CAD build for the part. Positions are in the model's coordinates, mm. A direction names the side the tool comes from. Coordinates: 2 decimals unless noted, no trailing zeros. Loops run counter-clockwise (first coordinate to the right, second up) from the corner with the lowest first, then second, coordinate; pieces in that order, holes last. Notation, with made-up numbers: (15, 12.5) -> (74, 12.5) arc R13 cw to (74, 28.5) -> close; hole circle Ø3 at (-23, -18). An arc over 180 degrees is marked (long way). Answer as a JSON object with one key per item and string values. Group by question number.
from build123d import *

# Parameters (mm, degrees)
F0_R          = 52.3474844596
F1_DEPTH      = 118.872
F2_W          = 198.6170932651
F2_H          = 132.2823390365
F3_DEPTH      = 95.25
F5_ANGLE_BACK = 90
F5_ANGLE      = 180


with BuildPart() as f1:
    # F0 (on Top) → F1 (new body)
    with BuildSketch(Plane.XY):
        Circle(F0_R)
    extrude(amount=F1_DEPTH)

    # F2 (on face) → F3 (join)
    with BuildSketch(Plane.XY.offset(118.872)):
        with Locations((5.5361129344, -8.6901672184)):
            Rectangle(F2_W, F2_H)
    extrude(amount=F3_DEPTH)

    # F4 (on face) → F5 (revolve)
    with BuildSketch(Plane.XY.offset(214.122), mode=Mode.PRIVATE) as f5_sk:
        with BuildLine():
            Line((0, -34.9537354881), (0, 34.9537354881))
            ThreePointArc((0, 34.9537354881), (-34.9537354881, 0), (0, -34.9537354881))
        make_face()
    revolve(f5_sk.sketch.rotate(Axis((0, 0, 214.122), (0, 1, 0)), -F5_ANGLE_BACK), axis=Axis((0, 0, 214.122), (0, 1, 0)), revolution_arc=F5_ANGLE)


solid = f1.part
Item 1: Flat gauge pins, fed straight in: P1, Ø10, axis at y = -40.5, z = 65, coming from the +X side; P2, Ø4, axis at x = -9, y = 15.5, coming from the +Z side; P3, Ø1, axis at x = -9.5, z = 60, coming from the -Y side. Where does each tip first touch, or does it go through?
Item 2: Band-saw the part on D-D, the plane y = -65.5. List the corners of the cut face in (x, z).
Item 3: Band-saw the part on A-A, the plane y = 0. List the corners of the cut face in (x, z).
Item 4: 3-axis set-ups, long thin cutter, end or side, ignore diameter. For faces 1 (the flat face through (104.845, -10, 166)), 2 (the flat face through (48, -22, 118.872)), 3 (the flat face through (0, 0, 228)): which of +Z, -Z, +X, -X, +Y, -Y reach the whole face in a straight line?
Item 5: Drill centre lines: L1, parallel to Z at x = 1, y = 50.5; L2, parallel to Y at x = -2, z = 104; L3, parallel to Z at x = 1, y = -66. Where is each one in solid material? Low to high.
Item 6: Band-saw the part on B-B, the plane x = 42. List the corners of the cut face in (y, z), and give its area (3 significant figures).
Item 7: Band-saw the part on C-C, the plane z = 75.5. List the corners of the cut face in (x, y).
Reply:
{
 "1": {"P1": "x = 38.47", "P2": "z = 245.24", "P3": "y = -51.57"},
 "2": {"outline": "(-93.77, 118.87) -> (104.84, 118.87) -> (104.84, 214.12) -> (-93.77, 214.12) -> close"},
 "3": {"outline": "(-93.77, 118.87) -> (-52.35, 118.87) -> (-52.35, 0) -> (52.35, 0) -> (52.35, 118.87) -> (104.84, 118.87) -> (104.84, 214.12) -> (0, 214.12) -> (0, 249.08) arc R34.95 ccw to (-34.95, 214.12) -> (-93.77, 214.12) -> close"},
 "4": {"face 1": "+Z, -Z, +X, +Y, -Y", "face 2": "-Z", "face 3": "+Z, +X, +Y, -Y"},
 "5": {"L1": "0 to 214.12", "L2": "-52.31 to 52.31", "L3": "118.87 to 214.12"},
 "6": {"outline": "(-74.83, 118.87) -> (-31.25, 118.87) -> (-31.25, 0) -> (31.25, 0) -> (31.25, 118.87) -> (57.45, 118.87) -> (57.45, 214.12) -> (-74.83, 214.12) -> close", "area": "20,000 mm²"},
 "7": {"outline": "circle Ø104.69 at (0, 0)"}
}
